Work out the finished part from the listing and answer in its coordinate system (mm). A direction names the side the tool comes from. Give positions to 0.01 mm unless a question says otherwise; leave off trailing zeros. Order: outer loops, then holes, each group sorted by start corner. A loop starts at its lowest first (then second) coordinate and runs counter-clockwise, first axis right, second up. Notation, with made-up numbers: (18.5, -37.75) - (38.5, -37.75) arc R29 cw to (38.5, -5.75) - close; hole circle Ø7 at (-30.5, 42.5). An arc over 180 degrees is marked (long way). Write each question's results on one line, items separated by ' | '.
from build123d import *

# Parameters (mm, degrees)
CROQUIS1_W              = 50.8
CROQUIS1_H              = 80
CROQUIS1_R              = 4
SALIENTE_EXTRUIR1_DEPTH = 12.7
CROQUIS2_R              = 10
CORTAR_EXTRUIR1_DEPTH   = 5
CROQUIS3_W              = 50.8
CROQUIS3_H              = 12.7
SALIENTE_EXTRUIR2_DEPTH = 10


with BuildPart() as part:
    # Croquis1 → Saliente-Extruir1 (new body)
    with BuildSketch(Plane.XY):
        Rectangle(CROQUIS1_W, CROQUIS1_H)
        with Locations((0, -20)):
            Circle(CROQUIS1_R, mode=Mode.SUBTRACT)
    extrude(amount=SALIENTE_EXTRUIR1_DEPTH)

    # Croquis2 → Cortar-Extruir1 (cut)
    with BuildSketch(Plane.XY.offset(12.7)):
        with Locations((0, -20)):
            Circle(CROQUIS2_R)
    extrude(amount=-CORTAR_EXTRUIR1_DEPTH, mode=Mode.SUBTRACT)

    # Croquis3 → Saliente-Extruir2 (add)
    with BuildSketch(Plane.XZ.offset(40)):
        with Locations((0, 6.35)):
            Rectangle(CROQUIS3_W, CROQUIS3_H)
    extrude(amount=SALIENTE_EXTRUIR2_DEPTH)


solid = part.part
1. Straight lines are drawn through the part: line 1 (Y direction, x = 0, z = 3); line 2 (X direction, y = -20, z = 5.25); line 3 (Y direction, x = 0, z = 10.15). For each, find the intervals that lie inside material, in ascending order. Write a range as [from, to].
Answer list:
line 1: [-50, -24], [-16, 40] | line 2: [-25.4, -4], [4, 25.4] | line 3: [-50, -30], [-10, 40]
2. A tool of negligible diameter and unlimited length cuts with its end or side. For faces 4 (the face through (-1.302, -10.085, 10.235)), 5 (the face through (-0.521, -16.034, 3.796)), from which of +Z, -Z, +X, -X, +Y, -Y can it reach the whole face along a straight path? Write none if from no direction.
Answer list:
face 4: +Z | face 5: +Z, -Z
3. A cutting plane is placed at B-B, the plane y = -20. Write down the section's boundary in (x, z).
Answer list:
outline: (-25.4, 0) - (-4, 0) - (-4, 7.7) - (-10, 7.7) - (-10, 12.7) - (-25.4, 12.7) - close; (4, 0) - (25.4, 0) - (25.4, 12.7) - (10, 12.7) - (10, 7.7) - (4, 7.7) - close
4. A cutting plane is placed at C-C, the plane z = 10. Write down the section's boundary in (x, y).
Answer list:
outline: (-25.4, -50) - (25.4, -50) - (25.4, 40) - (-25.4, 40) - close; hole circle Ø20 at (0, -20)
5. Determine the mould class of faces 1 (the face through (-0.1, -24.3, 7.7)), 2 (the face through (0, -4, 0)), 3 (the face through (-25.4, -4, 6)) for opening direction X: +X half, -X half, draft (parallel to the pull), parting line (faces both ways), or undercut.
Answer list:
face 1: undercut | face 2: draft | face 3: -X half
6. Given P1, Ø16, axis at x = 2, y = -15.5, coming from the +Z side; P2, Ø10.5, axis at x = 0, y = -20, coming from the +Z side, each flat-ended and moving along its own axis, determine where each tip first touches the part or whether it passes through.
Answer list:
P1: z = 12.7 | P2: z = 7.7
7. A cutting plane is placed at A-A, the plane x = 0. Write down the section's boundary in (y, z).
Answer list:
outline: (-50, 0) - (-24, 0) - (-24, 7.7) - (-30, 7.7) - (-30, 12.7) - (-50, 12.7) - close; (-16, 0) - (40, 0) - (40, 12.7) - (-10, 12.7) - (-10, 7.7) - (-16, 7.7) - close
